The listing builds one solid part. Answer for the finished solid, in the listing's coordinates (mm). Face numbers are marked on the shaded views. A direction names the side the tool comes from. Coordinates: 2 decimals unless noted, no trailing zeros. Order: outer loops, then holes, each group sorted by start corner. A loop starts at its lowest first (then second) coordinate and runs counter-clockwise, first axis right, second up. Notation, with made-up numbers: (38, 72) -> (89, 72) arc R35 ccw to (89, 104) -> close; hole circle Ø10 at (45, 84.25). An arc over 180 degrees is marked (long way). Write each question's results on one line, items separated by ' | '. Start each with the question number.
(1) Straight lines are drawn through the part: L1, parallel to Y at x = 60.5, z = 1; L2, parallel to X at y = 3, z = 12; L3, parallel to Y at x = 18.5, z = 0. For each, find the intervals that lie inside material, in ascending order.
(2) Given pin 1 (11 mm diameter, centred on y = 2.5, z = -9.5, fed in from +X); pin 2 (3 mm diameter, centred on y = 6.5, z = -7, fed in from -X); pin 3 (8 mm diameter, centred on y = 44.5, z = 0, fed in from -X), each flat-ended and moving along its own axis, determine where each tip first touches the part or whether it passes through.
(3) A tool of negligible diameter and unlimited length cuts with its end or side. For the marked faces 1, 2, 3 and 4, from which of +Z, -Z, +X, -X, +Y, -Y can it reach the whole face along a straight path? Write none if from no direction.
(4) The part is cut by section D-D, the plane z = -8.5. Give the vertices of the cut face in (x, y).
(5) The part is cut by section A-A, the plane z = -12.5. Give the vertices of the cut face in (x, y).
(6) The part is cut by section B-B, the plane y = 5.5. Give the vertices of the cut face in (x, z), then the cut area to 3 significant figures.
(7) The part is cut by section C-C, the plane x = 18. Give the vertices of the cut face in (y, z).
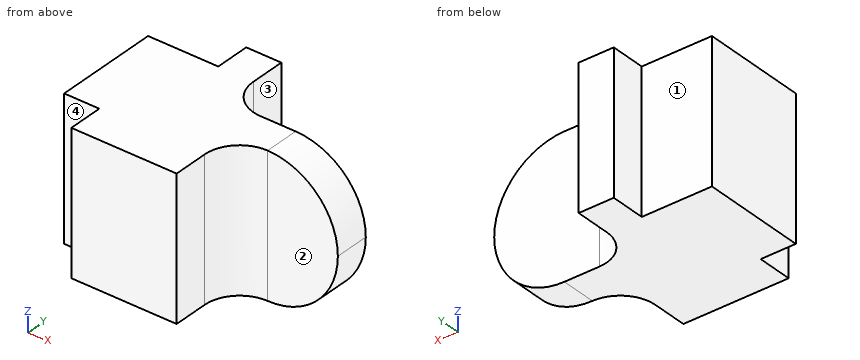
Autodesk Inventor part; units mm, degrees
ref_plane "YZ Plane" through (0, 0, 0) normal (1, 0, 0) x (0, 1, 0)
ref_plane "XZ Plane" through (0, 0, 0) normal (0, 1, 0) x (-1, 0, 0)
ref_plane "XY Plane" through (0, 0, 0) normal (0, 0, 1) x (1, 0, 0)
sketch "草圖1" plane through (0, 0, 0) normal (0, 0, 1) x (1, 0, 0)
  line L0 (0, 0) -> (0, 40)
  line L1 (0, 40) -> (20, 40)
  line L2 (20, 40) -> (20, 50)
  line L3 (20, 50) -> (30, 50)
  line L4 (30, 50) -> (30, 40)
  arc A0 (30, 40) -> (40, 30) centre (40, 40) ccw
  line L5 (40, 30) -> (70, 30)
  line L6 (70, 30) -> (70, 20)
  line L7 (70, 20) -> (50, 20)
  arc A1 (50, 20) -> (40, 10) centre (50, 10) ccw
  line L8 (40, 10) -> (40, 0)
  line L9 (40, 0) -> (0, 0)
  line L10 (0, 0) -> (10, 0)
  line L11 (10, 0) -> (10, 10)
  line L12 (10, 10) -> (0, 10)
  line L13 (0, 10) -> (0, 0)
  dimension "d0" = 40
  dimension "d1" = 20
  dimension "d2" = 10
  dimension "d3" = 50
  dimension "d4" = 70
  dimension "d5" = 40
  dimension "d6" = 10
  dimension "d7" = 20
  dimension "d8" = 10
  dimension "d9" = 10
  dimension "d10" = 10
extrude "擠出1" add sketch "草圖1" along normal mid plane 40 contours L0 L1 L2 L3 L4 A0 L5 L6 L7 A1 L8 L9 L11 L12
fillet "圓角1" radius 20 2 edges at (70, 25, 20) (70, 25, -20)
properties part number "21" material "鋼、碳鋼"
Established:
1) L1: y = 20 to 30 | L2: x = 10 to 40 | L3: y = 0 to 40
2) pin 1: stops at x = 40 | pin 2: stops at x = 10 | pin 3: stops at x = 20
3) face 1: +Z, -Z, -X, +Y | face 2: +Z, -Z, +X, -Y | face 3: +Z, -Z, +X, +Y | face 4: +Z, -Z, -X, -Y
4) outline: (0, 10) -> (10, 10) -> (10, 0) -> (40, 0) -> (40, 10) arc R10 cw to (50, 20) -> (68.1, 20) -> (68.1, 30) -> (40, 30) arc R10 cw to (30, 40) -> (30, 50) -> (20, 50) -> (20, 40) -> (0, 40) -> close
5) outline: (0, 10) -> (10, 10) -> (10, 0) -> (40, 0) -> (40, 10) arc R10 cw to (50, 20) -> (65.61, 20) -> (65.61, 30) -> (40, 30) arc R10 cw to (30, 40) -> (30, 50) -> (20, 50) -> (20, 40) -> (0, 40) -> close
6) outline: (10, -20) -> (40, -20) -> (40, 20) -> (10, 20) -> close | area: 1,200 mm^2
7) outline: (0, -20) -> (40, -20) -> (40, 20) -> (0, 20) -> close
